Here's how the part is built. I have some questions about the finished solid (model axes, mm). A direction names the side the tool comes from. Give positions to 0.01 mm unless a question says otherwise; leave off trailing zeros. Loops run counter-clockwise (first coordinate to the right, second up) from the corner with the lowest first, then second, coordinate; pieces in that order, holes last. Notation, with made-up numbers: (-34.75, -35.5) -> (20.25, -35.5) arc R19 cw to (20.25, -0.5) -> close; hole circle Ø8 at (74.5, 36). An arc over 180 degrees is marked (long way). Answer in a Markdown table with one row per item. Add a question column.
Item 1: If I drill on line 1 (Z direction, x = 1.45, y = 8.5); line 2 (Z direction, x = 0.9, y = 8.75); line 3 (Z direction, x = 1.5, y = 3.5), over which ranges is the centre line in solid material (lowest first)?
Item 2: For P1, Ø0.8, axis at x = 0.5, z = 5, coming from the -Y side; P2, Ø0.8, axis at x = 1, z = -3.5, coming from the +Y side; P3, Ø5.5, axis at y = 6.25, z = 7.26, coming from the -X side, each with a flat end and sliding along its axis, tell me the tip position at first contact or that it passes through.
Item 3: If we section it at A-A (x = 0.4): Write out the boundary of the cut face in (y, z).
Item 4: We'd pull the mould along Y, two halves only. Please class faces 4 (the face through (0.79, 9.37, 10.65)), 5 (the face through (1, 1, -10)), 6 (the face through (0.79, 4.42, -4.88)): released by +Y, released by -Y, zero draft, split by the parting line, or undercut.
Item 5: Which directions (+Z, -Z, +X, -X, +Y, -Y) give clear straight access to the entire face, cutting with the end or side of a thin tool? Please do faces 1 (the face through (1, 12, -9)), 2 (the face through (1, 1.8, 5)), 3 (the face through (1, 1, 10)).
Item 6: If we section it at C-C (z = 8.25): Write out the boundary of the cut face in (x, y).
Item 7: If we section it at B-B (y = 4.8): Write out the boundary of the cut face in (x, z).
Item 8: If we section it at D-D (y = 8.5): Write out the boundary of the cut face in (x, z).
```python
from build123d import *

# Parameters (mm, degrees)
SKETCH_2_R      = 3
EXTRUDE_1_DEPTH = 1.6


with BuildPart() as part:
    # 스케치2 → 보스-돌출1 (new body)
    with BuildSketch(Plane(origin=(0, 0, 0), x_dir=(0, 0, -1), z_dir=(1, 0, 0))):
        with BuildLine():
            Line((12, 1), (8, 1))
            Line((8, 1), (8, 1.8))
            Line((8, 1.8), (1.658312395, 1.8))
            Line((1.658312395, 1.8), (1.658312395, 2.3))
            ThreePointArc((1.658312395, 2.3), (0, 7.8), (-1.658312395, 2.3))
            Line((-1.658312395, 2.3), (-1.658312395, 1.8))
            Line((-1.658312395, 1.8), (-8, 1.8))
            Line((-8, 1.8), (-8, 1))
            Line((-8, 1), (-12, 1))
            Line((-12, 1), (-12, 6.056548766))
            ThreePointArc((-12, 6.056548766), (-10.6106753, 9.4106753), (-7.256548766, 10.8))
            Line((-7.256548766, 10.8), (9, 10.8))
            Line((9, 10.8), (9, 12.8))
            Line((9, 12.8), (12, 12.8))
            Line((12, 12.8), (12, 1))
        make_face()
        with Locations((-7.256548766, 6.25)):
            Circle(SKETCH_2_R, mode=Mode.SUBTRACT)
        with Locations((7.256548766, 6.25)):
            Circle(SKETCH_2_R, mode=Mode.SUBTRACT)
    extrude(amount=EXTRUDE_1_DEPTH)


solid = part.part
```
Recorded:
| question | item | result |
|---|---|---|
| 1 | line 1 | z = -12 to -9.24, -5.27 to 5.27, 9.24 to 11.32 |
| 1 | line 2 | z = -12 to -8.91, -5.6 to 5.6, 8.91 to 11.16 |
| 1 | line 3 | z = -12 to -8.46, -6.06 to -2.7, 2.7 to 6.06, 8.46 to 12 |
| 2 | P1 | stops at y = 1.8 |
| 2 | P2 | stops at y = 10.8 |
| 2 | P3 | passes through |
| 3 | outline | (1, -12) -> (12.8, -12) -> (12.8, -9) -> (10.8, -9) -> (10.8, 7.26) arc R4.74 ccw to (6.06, 12) -> (1, 12) -> (1, 8) -> (1.8, 8) -> (1.8, 1.66) -> (2.3, 1.66) arc R3 cw (long way) to (2.3, -1.66) -> (1.8, -1.66) -> (1.8, -8) -> (1, -8) -> close; hole circle Ø6 at (6.25, -7.26); hole circle Ø6 at (6.25, 7.26) |
| 4 | face 4 | released by +Y |
| 4 | face 5 | released by -Y |
| 4 | face 6 | undercut |
| 5 | face 1 | +Z, +X, -X, +Y |
| 5 | face 2 | +X, -X, -Y |
| 5 | face 3 | +Z, -Z, +X, -X, -Y |
| 6 | outline | (0, 1) -> (1.6, 1) -> (1.6, 3.42) -> (0, 3.42) -> close; (0, 9.08) -> (1.6, 9.08) -> (1.6, 10.69) -> (0, 10.69) -> close |
| 7 | outline | (0, -12) -> (1.6, -12) -> (1.6, -9.88) -> (0, -9.88) -> close; (0, -4.63) -> (1.6, -4.63) -> (1.6, -3) -> (0, -3) -> close; (0, 3) -> (1.6, 3) -> (1.6, 4.63) -> (0, 4.63) -> close; (0, 9.88) -> (1.6, 9.88) -> (1.6, 12) -> (0, 12) -> close |
| 8 | outline | (0, -12) -> (1.6, -12) -> (1.6, -9.24) -> (0, -9.24) -> close; (0, -5.27) -> (1.6, -5.27) -> (1.6, 5.27) -> (0, 5.27) -> close; (0, 9.24) -> (1.6, 9.24) -> (1.6, 11.32) -> (0, 11.32) -> close |
